Source: CAD feature listing. Evaluate the final solid. Frame: model axes, mm. A direction names the side the tool comes from. Give positions to 0.01 mm unless a question says otherwise; leave off trailing zeros. Write each loop counter-clockwise with the first axis right and the second up, starting at its lowest first coordinate (ties: lowest second). Pieces come first, ordered by that corner, then holes. Notation, with made-up numbers: M 20,56 L 32,56 A25 cw 32,80 Z; hole C -7.75,41 d2. An arc over 180 degrees is marked long. Use CSV: the item, a comma, the result in double quotes. Start each with the question number.
from build123d import *

# Parameters (mm, degrees)
F0_W     = 5.6
F0_H     = 5.6
F0_R     = 2
F1_DEPTH = 30
F2_W     = 5.6
F2_H     = 4.6
F2_R     = 1.5
F3_DEPTH = 12.2
F4_W     = 5.6
F4_H     = 4.6
F4_R     = 1.5
F5_DEPTH = 12.2


with BuildPart() as f1:
    # F0 (on Top) → F1 (new body)
    with BuildSketch(Plane.XY):
        Rectangle(F0_W, F0_H)
        Circle(F0_R, mode=Mode.SUBTRACT)
    extrude(amount=F1_DEPTH)

    # F2 (on face) → F3 (join)
    with BuildSketch(Plane.YZ.offset(2.8)):
        with Locations((0, 15)):
            Rectangle(F2_W, F2_H)
        with Locations((0, 15)):
            Circle(F2_R, mode=Mode.SUBTRACT)
    extrude(amount=F3_DEPTH)

    # F4 (on face) → F5 (join)
    with BuildSketch(Plane(origin=(-2.8, 0, 0), x_dir=(0, -1, 0), z_dir=(-1, 0, 0))):
        with Locations((0, 15)):
            Rectangle(F4_W, F4_H)
        with Locations((0, 15)):
            Circle(F4_R, mode=Mode.SUBTRACT)
    extrude(amount=F5_DEPTH)


solid = f1.part
1. Section B-B on x = 0. Return loops of the section in (y, z), then the cut area to 3 significant figures.
2. Line query: probe 1 along Z at (x, y) = (-6.25, 0); probe 2 along Y at (x, z) = (0, 14.5); probe 3 along X at (y, z) = (-1.8, 13.5). Output: solid intervals per line, ascending.
3. Section D-D on x = 3.25. Return loops of the section in (y, z).
4. Section C-C on y = 0. Return loops of the section in (x, z).
5. Section A-A on z = 22.5. Return loops of the section in (x, y), then the cut area to 3 significant figures.
6. First-contact query: pin 1 (2 mm diameter, centred on y = 0.5, z = 9, fed in from +X); pin 2 (3 mm diameter, centred on y = 1.5, z = 8.5, fed in from -X); pin 3 (1.7 mm diameter, centred on x = 7.5, y = -1, fed in from -Z). Flat tips, straight axial feed; report the tip coordinate or a pass-through.
7. Access query for faces 5 (the flat face through (2.8, 0, 15)), 6 (the flat face through (2.8, 0, 24)), 7 (the flat face through (-9, 0, 12.7)), 8 (the flat face through (9, 0, 12.7)), 9 (the flat face through (-2.8, 0, 24)). Directions: +Z, -Z, +X, -X, +Y, -Y. A direction counts if a zero-diameter tool reaches every point of the face in a straight line with its end or side. Return the directions, or none.
8. Pull-direction query (Z, two-part tool) for faces 1 (the flat face through (-2.8, 0, 15)), 2 (the cylindrical face through (8.81, -1.11, 16.01)), 3 (the flat face through (-1, 2, 0)), 4 (the flat face through (-15, 0, 17)); classes: released by +Z, released by -Z, zero draft, split by the parting line, or undercut.
Resolved:
1,outline,"M -2.8,0 L -2,0 L -2,30 L -2.8,30 Z; M 2,0 L 2.8,0 L 2.8,30 L 2,30 Z"
1,area,"48.0 mm2"
2,probe 1,"z = 12.7 to 13.5, 16.5 to 17.3"
2,probe 2,"y = -2.8 to -2, 2 to 2.8"
2,probe 3,"x = -15 to -0.87, 0.87 to 15"
3,outline,"M -2.8,12.7 L 2.8,12.7 L 2.8,17.3 L -2.8,17.3 Z; hole C 0,15 d3"
4,outline,"M -15,12.7 L -2.8,12.7 L -2.8,0 L -2,0 L -2,30 L -2.8,30 L -2.8,17.3 L -15,17.3 L -15,16.5 L -2.8,16.5 L -2.8,13.5 L -15,13.5 Z; M 2,0 L 2.8,0 L 2.8,12.7 L 15,12.7 L 15,13.5 L 2.8,13.5 L 2.8,16.5 L 15,16.5 L 15,17.3 L 2.8,17.3 L 2.8,30 L 2,30 Z"
5,outline,"M -2.8,-2.8 L 2.8,-2.8 L 2.8,2.8 L -2.8,2.8 Z; hole C 0,0 d4"
5,area,"18.8 mm2"
6,pin 1,"stops at x = 2.8"
6,pin 2,"stops at x = -2.8"
6,pin 3,"stops at z = 12.7"
7,face 5,"+X"
7,face 6,"+Z, +X, +Y, -Y"
7,face 7,"-Z, -X, +Y, -Y"
7,face 8,"-Z, +X, +Y, -Y"
7,face 9,"+Z, -X, +Y, -Y"
8,face 1,"undercut"
8,face 2,"undercut"
8,face 3,"released by -Z"
8,face 4,"zero draft"
